Check sheet for the modelled part. Datum: model origin and axes. Units: mm. Face numbers are marked on the shaded views. A direction names the side the tool comes from. Round coordinates to 2 decimals unless told otherwise and drop trailing zeros. Order: outer loops, then holes, each group sorted by start corner. A loop starts at its lowest first (then second) coordinate and runs counter-clockwise, first axis right, second up. Notation, with made-up numbers: (-10, 44) -> (22, 44) arc R7 cw to (22, 50) -> close; hole circle Ø1 at (27, -13.75). An arc over 180 degrees is marked (long way). Answer as CSV lines item,"result". Start each with the question number.
from build123d import *

# Parameters (mm, degrees)
F0_W     = 807.72
F0_H     = 401.32
F1_DEPTH = 243.84
F2_R     = 60.96
F3_DEPTH = 45.72
F4_W     = 746.76
F4_H     = 340.36
F4_R     = 82.55
F4_R_2   = 60.96
F5_DEPTH = 213.36


with BuildPart() as f1:
    # F0 (on Top) → F1 (new body)
    with BuildSketch(Plane.XY):
        with Locations((-9.350765, -16.714708)):
            Rectangle(F0_W, F0_H)
    extrude(amount=F1_DEPTH)

    # F2 (on face) → F3 (join)
    with BuildSketch(Plane.XY.offset(243.84)):
        with Locations((-314.150765, 84.885292)):
            Circle(F2_R)
        with Locations((-314.150765, -118.314708)):
            Circle(F2_R)
        with Locations((-110.950765, 84.885292)):
            Circle(F2_R)
        with Locations((92.249235, 84.885292)):
            Circle(F2_R)
        with Locations((92.249235, -118.314708)):
            Circle(F2_R)
        with Locations((-110.950765, -118.314708)):
            Circle(F2_R)
        with Locations((295.449235, 84.885292)):
            Circle(F2_R)
        with Locations((295.449235, -118.314708)):
            Circle(F2_R)
    extrude(amount=F3_DEPTH)

    # F4 (on face) → F5 (cut)
    with BuildSketch(Plane(origin=(0, 0, 0), x_dir=(1, 0, 0), z_dir=(0, 0, -1))):
        with Locations((-9.350765, 16.714708)):
            Rectangle(F4_W, F4_H)
        with Locations((-212.550765, 16.714708)):
            Circle(F4_R, mode=Mode.SUBTRACT)
        with Locations((-9.350765, 16.714708)):
            Circle(F4_R, mode=Mode.SUBTRACT)
        with Locations((193.849235, 16.714708)):
            Circle(F4_R, mode=Mode.SUBTRACT)
        with Locations((-212.550765, 16.714708)):
            Circle(F4_R_2)
        with Locations((-9.350765, 16.714708)):
            Circle(F4_R_2)
        with Locations((193.849235, 16.714708)):
            Circle(F4_R_2)
    extrude(amount=-F5_DEPTH, mode=Mode.SUBTRACT)


solid = f1.part
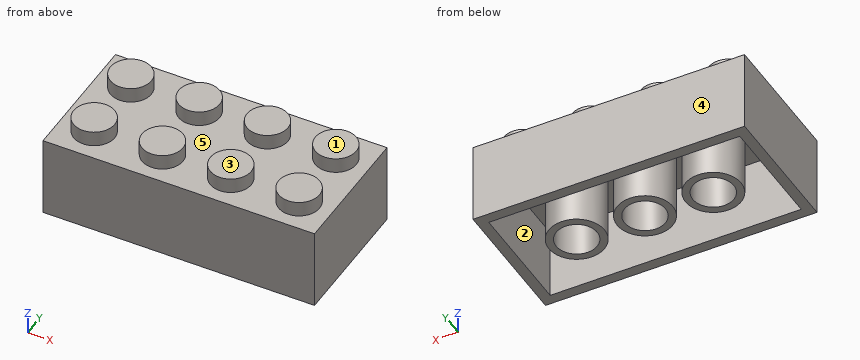
1) Section check D-D on y = -136. Record the cut outline in (x, z), then the cut area to 3 significant figures.
2) Depth check by flat-ended pin: pin 1 Ø4 at (x, y) = (54, -67) entering from +Z; pin 2 Ø10 at (x, y) = (295.5, -173) entering from -Z. Enter the tip coordinate at first touch or a pass-through.
3) Mould release check, pull along Y, two halves, no side actions. Record for the marked faces 3, 4 and 5: released by +Y, released by -Y, zero draft, split by the parting line, or undercut.
4) Section check A-A on z = 42. Record the cut outline in (x, y), then the cut area to 3 significant figures.
5) Material ranges on line 1 along Y through (x, z) = (-213, 25); line 2 along X through (y, z) = (151, 118.5); line 3 along Y through (x, z) = (-285, 91), recorded low to high.
6) Section check C-C on x = -306.5. Record the cut outline in (y, z).
7) Access from +Z, -Z, +X, -X, +Y, -Y to the whole of each face (thin tool, end or side, straight path). Record for the marked faces 1 and 2.
Solutions:
1,outline,"(-413.21, 0) -> (-382.73, 0) -> (-382.73, 213.36) -> (364.03, 213.36) -> (364.03, 0) -> (394.51, 0) -> (394.51, 243.84) -> (353.79, 243.84) -> (353.79, 289.56) -> (237.11, 289.56) -> (237.11, 243.84) -> (150.59, 243.84) -> (150.59, 289.56) -> (33.91, 289.56) -> (33.91, 243.84) -> (-52.61, 243.84) -> (-52.61, 289.56) -> (-169.29, 289.56) -> (-169.29, 243.84) -> (-255.81, 243.84) -> (-255.81, 289.56) -> (-372.49, 289.56) -> (-372.49, 243.84) -> (-413.21, 243.84) -> close"
1,area,"59,000 mm^2"
2,pin 1,"stops at z = 243.84"
2,pin 2,"stops at z = 213.36"
3,face 3,"zero draft"
3,face 4,"released by +Y"
3,face 5,"undercut"
4,outline,"(-413.21, -217.37) -> (394.51, -217.37) -> (394.51, 183.95) -> (-413.21, 183.95) -> close; circle Ø165.1 at (-212.55, -16.71); circle Ø165.1 at (-9.35, -16.71); circle Ø165.1 at (193.85, -16.71); hole (-382.73, -186.89) -> (364.03, -186.89) -> (364.03, 153.47) -> (-382.73, 153.47) -> close; hole circle Ø121.92 at (-212.55, -16.71); hole circle Ø121.92 at (-9.35, -16.71); hole circle Ø121.92 at (193.85, -16.71)"
4,area,"99,200 mm^2"
5,line 1,"y = -217.37 to -186.89, -99.26 to -77.67, 44.24 to 65.83, 153.47 to 183.95"
5,line 2,"x = -413.21 to -382.73, 364.03 to 394.51"
5,line 3,"y = -217.37 to -186.89, -56.28 to 22.85, 153.47 to 183.95"
6,outline,"(-217.37, 0) -> (-186.89, 0) -> (-186.89, 213.36) -> (153.47, 213.36) -> (153.47, 0) -> (183.95, 0) -> (183.95, 243.84) -> (145.36, 243.84) -> (145.36, 289.56) -> (24.41, 289.56) -> (24.41, 243.84) -> (-57.84, 243.84) -> (-57.84, 289.56) -> (-178.79, 289.56) -> (-178.79, 243.84) -> (-217.37, 243.84) -> close"
7,face 1,"+Z, +X, -X, +Y, -Y"
7,face 2,"-Z"
